```python
from build123d import *

# Parameters (mm, degrees)
SKETCH_1_W          = 106.172
SKETCH_1_H          = 32.7
SKETCH_1_R          = 1.778
EXTRUDE_1_DEPTH     = 15
SKETCH_2_W          = 106.172
SKETCH_2_H          = 32.7
SKETCH_2_R          = 1.778
EXTRUDE_2_DEPTH     = 30
EXTRUDE_3_DEPTH     = 106
SKETCH_8_W          = 106.172
SKETCH_8_H          = 7.597957824
EXTRUDE_5_DEPTH     = 140
CUT_EXTRUDE_1_DEPTH = 146
SKETCH_11_W         = 106.172
SKETCH_11_H         = 7.597957824
EXTRUDE_7_DEPTH     = 10
SKETCH_15_W         = 106.17086593
SKETCH_15_H         = 5
EXTRUDE_11_DEPTH    = 60
SKETCH_16_W         = 18
SKETCH_16_H         = 12
CUT_EXTRUDE_2_DEPTH = 7.8
SKETCH_18_R         = 1.875
CUT_EXTRUDE_3_DEPTH = 10
SKETCH_20_W         = 106.172
SKETCH_20_H         = 22.709616495
CUT_EXTRUDE_4_DEPTH = 33
SKETCH_21_W         = 106.172
SKETCH_21_H         = 22.709616495
CUT_EXTRUDE_5_DEPTH = 5
SKETCH_30_W         = 62.094803524
SKETCH_30_H         = 19.778637262
CUT_EXTRUDE_6_DEPTH = 10


with BuildPart() as part:
    # 스케치1 → 보스-돌출1 (new body)
    with BuildSketch(Plane.XY):
        with Locations((3.3528, 15.362172506)):
            Rectangle(SKETCH_1_W, SKETCH_1_H)
        with Locations((46.0248, 11.812172506)):
            Circle(SKETCH_1_R, mode=Mode.SUBTRACT)
        with Locations((34.8488, 11.812172506)):
            Circle(SKETCH_1_R, mode=Mode.SUBTRACT)
        with Locations((-38.7332, 12.012172506)):
            Circle(SKETCH_1_R, mode=Mode.SUBTRACT)
        with Locations((-27.5332, 12.012172506)):
            Circle(SKETCH_1_R, mode=Mode.SUBTRACT)
    extrude(amount=EXTRUDE_1_DEPTH)

    # 스케치2 → 보스-돌출2 (add)
    with BuildSketch(Plane.XY.offset(15)):
        with Locations((3.3528, 15.362172506)):
            Rectangle(SKETCH_2_W, SKETCH_2_H)
        with Locations((-38.7332, 12.012172506)):
            Circle(SKETCH_2_R, mode=Mode.SUBTRACT)
        with Locations((-27.5332, 12.012172506)):
            Circle(SKETCH_2_R, mode=Mode.SUBTRACT)
        with Locations((34.8488, 11.812172506)):
            Circle(SKETCH_2_R, mode=Mode.SUBTRACT)
        with Locations((46.0248, 11.812172506)):
            Circle(SKETCH_2_R, mode=Mode.SUBTRACT)
    extrude(amount=EXTRUDE_2_DEPTH)

    # 스케치4 → 보스-돌출3 (add)
    with BuildSketch(Plane.ZY.offset(49.7332)):
        Polygon((45, -0.987827494), (25.502768184, 31.712172506), (45, 31.712172506), align=None)
    extrude(amount=-EXTRUDE_3_DEPTH)

    # 스케치8 → 보스-돌출5 (add)
    with BuildSketch(Plane(origin=(0, 31.712172506, 0), x_dir=(1, 0, 0), z_dir=(0, 1, 0))):
        with Locations((3.3528, -41.201021088)):
            Rectangle(SKETCH_8_W, SKETCH_8_H)
    extrude(amount=EXTRUDE_5_DEPTH)

    # 스케치9 → 컷-돌출1 (cut)
    with BuildSketch(Plane.ZY.offset(49.7332)):
        Polygon((45, -0.987827494), (17.051243473, -0.987827494), (45, 21.721789001), align=None)
    extrude(amount=-CUT_EXTRUDE_1_DEPTH, mode=Mode.SUBTRACT)

    # 스케치11 → 보스-돌출7 (add)
    with BuildSketch(Plane(origin=(0, 171.712172506, 0), x_dir=(1, 0, 0), z_dir=(0, 1, 0))):
        with Locations((3.3528, -41.201021088)):
            Rectangle(SKETCH_11_W, SKETCH_11_H)
    extrude(amount=EXTRUDE_7_DEPTH)

    # 스케치15 → 보스-돌출11 (add)
    with BuildSketch(Plane(origin=(0, 0, 37.402042176), x_dir=(-1, 0, 0), z_dir=(0, 0, -1))):
        with Locations((-3.352232965, 179.212172506)):
            Rectangle(SKETCH_15_W, SKETCH_15_H)
    extrude(amount=EXTRUDE_11_DEPTH)

    # 스케치16 → 컷-돌출2 (cut)
    with BuildSketch(Plane.XY.offset(45)):
        with Locations((3.3528, 43.784089849)):
            Rectangle(SKETCH_16_W, SKETCH_16_H)
    extrude(amount=-CUT_EXTRUDE_2_DEPTH, mode=Mode.SUBTRACT)

    # 스케치18 → 컷-돌출3 (cut)
    with BuildSketch(Plane.XY.offset(45)):
        with Locations((-13.882118572, 128.141421182)):
            Circle(SKETCH_18_R)
        with Locations((21.515537396, 124.701234261)):
            Circle(SKETCH_18_R)
        with Locations((0.28811198, 95.127423383)):
            Circle(SKETCH_18_R)
    extrude(amount=-CUT_EXTRUDE_3_DEPTH, mode=Mode.SUBTRACT)

    # 스케치20 → 컷-돌출4 (cut)
    with BuildSketch(Plane.XY.offset(45)):
        with Locations((3.3528, 10.366980754)):
            Rectangle(SKETCH_20_W, SKETCH_20_H)
    extrude(amount=-CUT_EXTRUDE_4_DEPTH, mode=Mode.SUBTRACT)

    # 스케치21 → 컷-돌출5 (cut)
    with BuildSketch(Plane.XY.offset(12)):
        with Locations((3.3528, 10.366980754)):
            Rectangle(SKETCH_21_W, SKETCH_21_H)
    extrude(amount=-CUT_EXTRUDE_5_DEPTH, mode=Mode.SUBTRACT)

    # 스케치30 → 컷-돌출6 (cut)
    with BuildSketch(Plane.XY.offset(45)):
        with Locations((3.3528, 152.636415487)):
            Rectangle(SKETCH_30_W, SKETCH_30_H)
    extrude(amount=-CUT_EXTRUDE_6_DEPTH, mode=Mode.SUBTRACT)


solid = part.part
```
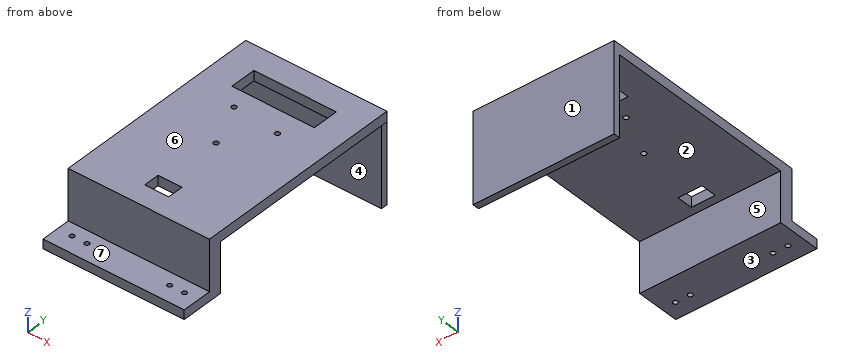
Here's how the part is built. I have some questions about the finished solid (model axes, mm). Face numbers are marked on the shaded views. A direction names the side the tool comes from. Coordinates: 2 decimals unless noted, no trailing zeros. Order: outer loops, then holes, each group sorted by start corner. A loop starts at its lowest first (then second) coordinate and runs counter-clockwise, first axis right, second up.
Item 1: Thinking about a two-plate mould opening in Y: for the marked faces 1, 2, 3 and 4, which applies, pulls with the +Y half, pulls with the -Y half, needs draft (parallel to the pull), parting line crosses it, or undercut?
Response values:
face 1: pulls with the +Y half
face 2: undercut
face 3: needs draft
face 4: undercut
Item 2: I'm going to push flat-ended pins straight in: pin 1 Ø4.5 at (x, y) = (21.52, 124.7) entering from -Z; pin 2 Ø1.5 at (x, z) = (-3.5, 8.5) entering from -Y; pin 3 Ø18 at (x, z) = (-19, 9) entering from -Y; pin 4 Ø5.5 at (x, y) = (-38.73, 12.01) entering from +Z. Where does each tip first touch, or does it pass through?
Response values:
pin 1: stops at z = 37.4
pin 2: stops at y = 21.72
pin 3: stops at y = -0.99
pin 4: stops at z = 7
Item 3: If we section it at D-D, the plane z = -12: List the corners of the cut face in (x, y) for me.
Response values:
outline: (-49.73, 176.71) - (56.44, 176.71) - (56.44, 181.71) - (-49.73, 181.71) - close
Item 4: If we section it at B-B, the plane x = -22: List the corners of the cut face in (y, z) for me.
Response values:
outline: (-0.99, 0) - (31.71, 0) - (31.71, 37.4) - (142.75, 37.4) - (142.75, 45) - (21.72, 45) - (21.72, 7) - (-0.99, 7) - close; (162.53, 37.4) - (176.71, 37.4) - (176.71, -22.6) - (181.71, -22.6) - (181.71, 45) - (162.53, 45) - close
Item 5: If we section it at C-C, the plane z = 25: List the corners of the cut face in (x, y) for me.
Response values:
outline: (-49.73, 21.72) - (56.44, 21.72) - (56.44, 31.71) - (-49.73, 31.71) - close; (-49.73, 176.71) - (56.44, 176.71) - (56.44, 181.71) - (-49.73, 181.71) - close
Item 6: I need wall thicknesses on probe 1 along Y at (x, z) = (-4, 33); probe 2 along Y at (x, z) = (-33, 5.5); probe 3 along Z at (x, y) = (-25.5, 132.5). Which ranges of each line are inside material? Lowest first, please.
Response values:
probe 1: y = 21.72 to 31.71, 176.71 to 181.71
probe 2: y = -0.99 to 31.71, 176.71 to 181.71
probe 3: z = 37.4 to 45
Item 7: If we section it at A-A, the plane y = 159.5: List the corners of the cut face in (x, z) for me, then the cut area to 3 significant figures.
Response values:
outline: (-49.73, 37.4) - (-27.69, 37.4) - (-27.69, 45) - (-49.73, 45) - close; (34.4, 37.4) - (56.44, 37.4) - (56.44, 45) - (34.4, 45) - close
area: 335 mm2
Item 8: Which directions (+Z, -Z, +X, -X, +Y, -Y) give clear straight access to the entire face, cutting with the end or side of a thin tool? Please do the marked faces 5, 6 and 7.
Response values:
face 5: -Z, +X, -X
face 6: +Z, +X, -X, +Y, -Y
face 7: +Z, +X, -X, -Y
